Here's the drawing with two shaded views (mm, measured from the low corner). I have some questions. A direction names the side the tool comes from. Coordinates: 2 decimals unless noted, no trailing zeros. Order: outer loops, then holes, each group sorted by start corner. A loop starts at its lowest first (then second) coordinate and runs counter-clockwise, first axis right, second up. Notation, with made-up numbers: (-23.5, -22.75) -> (2.5, -22.75) arc R33 ccw to (2.5, 11.25) -> close; hole circle Ø6 at (40, -38). An arc over 180 degrees is marked (long way). Answer as a JSON object with one key per item and string values. Group by question number.
(1) I want a section at D-D, the plane y = 12. List the corners of the cut face in (x, z) for me, plus the area to 3 significant figures.
(2) For pin 1 (8 mm diameter, centred on x = 21.5, z = 12.5, fed in from -Y); pin 2 (4 mm diameter, centred on y = 10, z = 16, fed in from +X); pin 3 (1.5 mm diameter, centred on x = 28.5, y = 10, fed in from +Z); pin 4 (4 mm diameter, centred on y = 7.5, z = 14.5, fed in from -X), each with a flat end and sliding along its axis, tell me the tip position at first contact or that it passes through.
(3) I need wall thicknesses on line 1 (X direction, y = 14, z = 14); line 2 (Z direction, x = 15, y = 9.75); line 3 (Y direction, x = 27.5, z = 3.5). Which ranges of each line are inside material? Lowest first, please.
(4) I want a section at B-B, the plane y = 8.75. List the corners of the cut face in (x, z) for me.
(5) I want a section at C-C, the plane z = 2.75. List the corners of the cut face in (x, y) for me.
(6) I want a section at A-A, the plane x = 15. List the corners of the cut face in (y, z) for me, plus the area to 3 significant figures.
(7) Which directions (+Z, -Z, +X, -X, +Y, -Y) give clear straight access to the entire face, cutting with the end or side of a thin tool? Please do the marked faces 1, 2 and 3.
(8) If we mould it in two halves opening along Z, with no side actions, what happens to the marked faces 4, 5 and 6? For each: pulls with the +Z half, pulls with the -Z half, needs draft (parallel to the pull), parting line crosses it, or undercut.
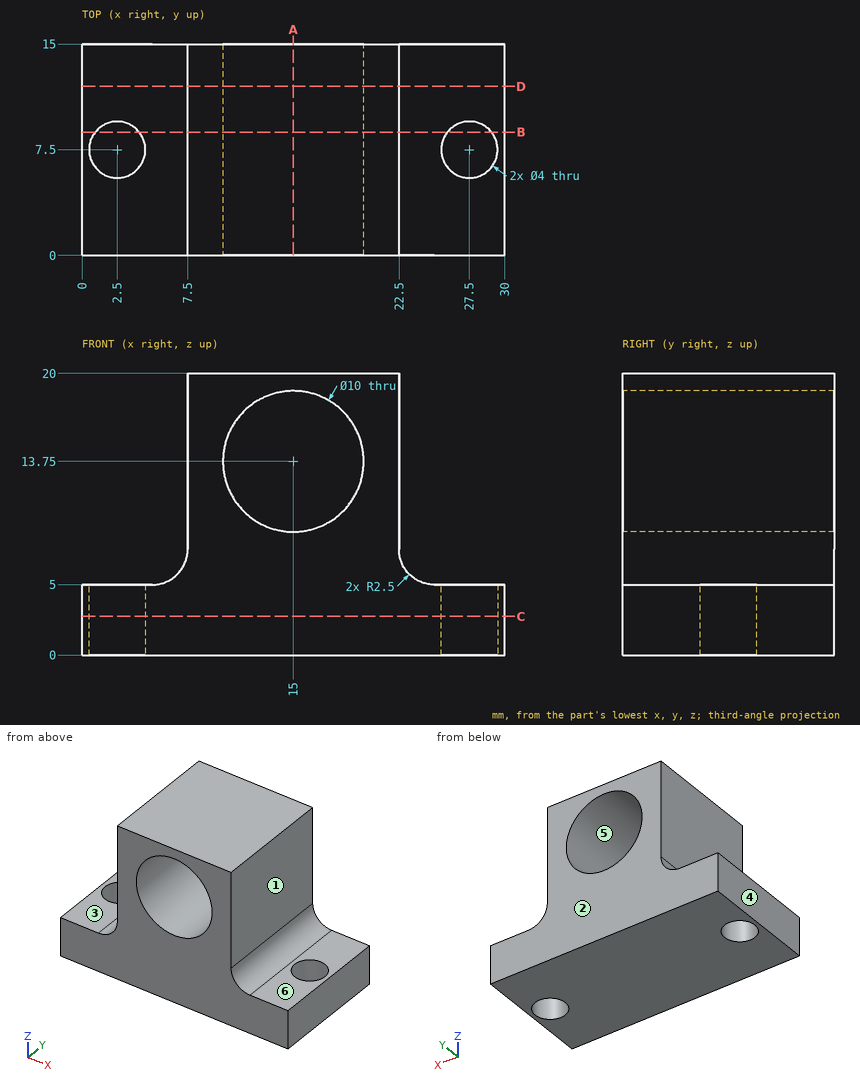
Computed values:
{
 "1": {"outline": "(0, 0) -> (30, 0) -> (30, 5) -> (25, 5) arc R2.5 cw to (22.5, 7.5) -> (22.5, 20) -> (7.5, 20) -> (7.5, 7.5) arc R2.5 cw to (5, 5) -> (0, 5) -> close; hole circle Ø10 at (15, 13.75)", "area": "299 mm2"},
 "2": {"pin 1": "stops at y = 0", "pin 2": "stops at x = 22.5", "pin 3": "stops at z = 5", "pin 4": "stops at x = 7.5"},
 "3": {"line 1": "x = 7.5 to 10.01, 19.99 to 22.5", "line 2": "z = 0 to 8.75, 18.75 to 20", "line 3": "y = 0 to 5.5, 9.5 to 15"},
 "4": {"outline": "(0, 0) -> (0.94, 0) -> (0.94, 5) -> (0, 5) -> close; (4.06, 0) -> (25.94, 0) -> (25.94, 5) -> (25, 5) arc R2.5 cw to (22.5, 7.5) -> (22.5, 20) -> (7.5, 20) -> (7.5, 7.5) arc R2.5 cw to (5, 5) -> (4.06, 5) -> close; (29.06, 0) -> (30, 0) -> (30, 5) -> (29.06, 5) -> close; hole circle Ø10 at (15, 13.75)"},
 "5": {"outline": "(0, 0) -> (30, 0) -> (30, 15) -> (0, 15) -> close; hole circle Ø4 at (2.5, 7.5); hole circle Ø4 at (27.5, 7.5)"},
 "6": {"outline": "(0, 0) -> (15, 0) -> (15, 8.75) -> (0, 8.75) -> close; (0, 18.75) -> (15, 18.75) -> (15, 20) -> (0, 20) -> close", "area": "150 mm2"},
 "7": {"face 1": "+Z, +X, +Y, -Y", "face 2": "+Z, -Z, +X, -X, +Y", "face 3": "+Z, -X, +Y, -Y"},
 "8": {"face 4": "needs draft", "face 5": "undercut", "face 6": "pulls with the +Z half"}
}
